The model under review builds one solid part; all positions refer to its coordinate system, in mm. Face numbers are marked on the shaded views. A direction names the side the tool comes from. Coordinates: 2 decimals unless noted, no trailing zeros. Write each loop counter-clockwise with the first axis right and the second up, starting at its lowest first coordinate (ties: lowest second). Pieces come first, ordered by that corner, then holes.
Autodesk Inventor part; units mm, degrees
ref_plane "YZ Plane" through (0, 0, 0) normal (1, 0, 0) x (0, 1, 0)
ref_plane "XZ Plane" through (0, 0, 0) normal (0, 1, 0) x (-1, 0, 0)
ref_plane "XY Plane" through (0, 0, 0) normal (0, 0, 1) x (1, 0, 0)
sketch "스케치1" plane through (0, 0, 0) normal (0, 0, 1) x (1, 0, 0)
  circle A0 centre (-5.4019, -4.5) radius 1.35
  circle A1 centre (5.4019, -4.5) radius 1.35
  circle A2 centre (-10.2056, -4.5) radius 1.35
  circle A3 centre (10.2056, -4.5) radius 1.35
  line L0 (-3.0587, -2.4) -> (-3.0587, -6.5)
  arc A4 (-3.0587, -6.5) -> (-4.0587, -7.5) centre (-3.0587, -7.5) ccw
  line L1 (-4.0587, -7.5) -> (-12.6075, -7.5)
  line L2 (-12.6075, -7.5) -> (-12.6075, 7.5)
  line L3 (-12.6075, 7.5) -> (-17.6, 13.3735)
  line L4 (-17.6, 13.3735) -> (-17.6, 24.9)
  line L5 (-17.6, 24.9) -> (-12.2, 24.9)
  line L6 (-12.2, 24.9) -> (-12.2, 14.7038)
  arc A5 (-12.2, 14.7038) -> (-10.2, 12.7038) centre (-10.2, 14.7038) ccw
  line L7 (-10.2, 12.7038) -> (0, 12.7038)
  line L8 (0, 12.7038) -> (5.5223, 12.4914)
  line L9 (5.5223, 12.4914) -> (10.5959, 12.4914)
  arc A6 (10.5959, 12.4914) -> (12.5959, 14.4914) centre (10.5959, 14.4914) ccw
  line L10 (12.5959, 14.4914) -> (12.5959, 24.9)
  line L11 (12.5959, 24.9) -> (17.6, 24.9)
  line L12 (17.6, 24.9) -> (17.6, 13.3735)
  line L13 (17.6, 13.3735) -> (12.6075, 7.5)
  line L14 (12.6075, 7.5) -> (12.6075, -7.5)
  line L15 (12.6075, -7.5) -> (4.1413, -7.5)
  arc A7 (4.1413, -7.5) -> (3.1413, -6.5) centre (3.1413, -7.5) ccw
  line L16 (3.1413, -6.5) -> (3.1413, -2.4)
  arc A8 (3.1413, -2.4) -> (2.1413, -1.4) centre (3.1413, -1.4) ccw
  line L17 (2.1413, -1.4) -> (-2.0587, -1.4)
  arc A9 (-2.0587, -1.4) -> (-3.0587, -2.4) centre (-3.0587, -1.4) ccw
  circle A10 centre (-8.5, 10.1) radius 1.45
  circle A11 centre (-15, 16.4) radius 1.45
  circle A12 centre (15, 16.4) radius 1.45
  circle A13 centre (8.5, 10.1) radius 1.45
  line L18 (12.6075, -7.5) -> (-12.6075, -7.5)
  line L19 (-12.6075, -7.5) -> (-12.6075, -1.5)
  line L20 (-12.6075, -1.5) -> (12.6075, -1.5)
  line L21 (12.6075, -1.5) -> (12.6075, -7.5)
  line L22 (3.1413, -1.4) -> (3.0413, -1.4)
  line L23 (3.0413, -1.4) -> (3.0413, -1.5)
  line L24 (3.0413, -1.5) -> (3.1413, -1.5)
  line L25 (3.1413, -1.5) -> (3.1413, -1.4)
  line L26 (3.0413, -1.5) -> (-2.9587, -1.5)
  line L27 (-2.9587, -1.5) -> (-2.9587, -7.5)
  line L28 (-2.9587, -7.5) -> (3.0413, -7.5)
  line L29 (3.0413, -7.5) -> (3.0413, -1.5)
  point P0 (0, 0)
  point P1 (12.6075, -1.5)
  dimension "d0" = 6
  dimension "d1" = 0.1
  dimension "d2" = 0.1
  dimension "d3" = 6
  dimension "d4" = 6
extrude "돌출1" add sketch "스케치1" along normal blind 30 contours A9 L20 L27 L18 A4 L0 | L0 A4 L1 L2 L20 A9 | L20 L29 L18 L27 | L20 A8 L16 A7 L18 L29 | L20 L14 L15 A7 L16 A8
sketch "스케치3" plane through (-12.6075, -7.5, 0) normal (0, -1, 0) x (1, 0, 0)
  line L0 (15.7488, 36) -> (15.7488, 30)
  line L1 (9.5488, 36) -> (9.5488, 30)
  line L2 (15.7488, 36) -> (15.6488, 36)
  line L3 (15.6488, 36) -> (15.6488, 35.9)
  line L4 (15.6488, 35.9) -> (15.7488, 35.9)
  line L5 (15.7488, 35.9) -> (15.7488, 36)
  line L6 (15.6488, 35.9) -> (9.6488, 35.9)
  line L7 (9.6488, 35.9) -> (9.6488, 29.9)
  line L8 (9.6488, 29.9) -> (15.6488, 29.9)
  line L9 (15.6488, 29.9) -> (15.6488, 35.9)
  line L10 (15.6488, 35.9) -> (9.6488, 35.9)
  line L11 (9.6488, 35.9) -> (9.6488, 36)
  line L12 (9.6488, 36) -> (15.6488, 36)
  line L13 (15.6488, 36) -> (15.6488, 35.9)
  line L14 (0, 30) -> (25.215, 30)
  line L15 (0, 0) -> (0, 30)
  line L16 (0, 15) -> (25.215, 15)
  line L17 (25.215, 0) -> (25.215, 30)
  line L18 (15.7488, -6) -> (15.7488, 0)
  line L19 (9.5488, -6) -> (9.5488, 0)
  line L20 (15.7488, -6) -> (15.6488, -6)
  line L21 (15.6488, -6) -> (15.6488, -5.9)
  line L22 (15.6488, -5.9) -> (15.7488, -5.9)
  line L23 (15.7488, -5.9) -> (15.7488, -6)
  line L24 (15.6488, -5.9) -> (9.6488, -5.9)
  line L25 (9.6488, -5.9) -> (9.6488, 0.1)
  line L26 (9.6488, 0.1) -> (15.6488, 0.1)
  line L27 (15.6488, 0.1) -> (15.6488, -5.9)
  line L28 (15.6488, -5.9) -> (9.6488, -5.9)
  line L29 (9.6488, -5.9) -> (9.6488, -6)
  line L30 (9.6488, -6) -> (15.6488, -6)
  line L31 (15.6488, -6) -> (15.6488, -5.9)
  line L32 (0, 0) -> (25.215, 0)
  point P0 (12.6075, 0)
  dimension "d11" = 0.1
  dimension "d12" = 0.1
  dimension "d13" = 6
  dimension "d14" = 6
extrude "돌출2" add sketch "스케치3" against normal blind 6 contours L9 L14 L7 L6 | L9 L8 L7 L14 | L32 L25 L26 L27 | L27 L24 L25 L32 | L21 L30 L29 L24
sketch "스케치7" plane through (-12.6075, -7.5, 0) normal (0, -1, 0) x (1, 0, 0)
  line L0 (0, 30) -> (9.6488, 30)
  line L1 (0, 0) -> (0, 30)
  line L2 (0, 0) -> (9.6488, 0)
  line L3 (9.6488, 0) -> (9.6488, -6)
  line L4 (9.6488, -6) -> (15.6488, -6)
  line L5 (15.6488, -6) -> (15.6488, 0)
  line L6 (15.6488, 0) -> (25.215, 0)
  line L7 (25.215, 0) -> (25.215, 30)
  line L8 (15.6488, 30) -> (25.215, 30)
  line L9 (15.6488, 30) -> (15.6488, 35.9)
  line L10 (15.6488, 35.9) -> (9.6488, 35.9)
  line L11 (9.6488, 35.9) -> (9.6488, 30)
  line L12 (0, 0) -> (0, 30)
  line L13 (0, 0) -> (-2.3925, 0)
  line L14 (-2.3925, 0) -> (-2.3925, 30)
  line L15 (-2.3925, 30) -> (0, 30)
  line L16 (0, 30) -> (0, 0)
  line L17 (12.6075, 0) -> (12.6075, 30)
  line L18 (25.215, 0) -> (25.215, 30)
  line L19 (25.215, 0) -> (25.215, 30)
  line L20 (25.215, 0) -> (27.6075, 0)
  line L21 (27.6075, 0) -> (27.6075, 30)
  line L22 (27.6075, 30) -> (25.215, 30)
  line L23 (25.215, 30) -> (25.215, 0)
  dimension "d26" = 2.3925
extrude "돌출6" add sketch "스케치7" against normal blind 6 contours L1 L13 L14 L15 | L22 L21 L20 L7
sketch "스케치8" plane through (-15, -7.5, 0) normal (-1, 0, 0) x (0, 0, 1)
  line L0 (0, 0) -> (30, 0)
  line L1 (15, 0) -> (15, 6)
  line L2 (30, 6) -> (0, 6)
  line L3 (15, 6) -> (12, 6)
  line L4 (12, 6) -> (12, 0)
  line L5 (12, 0) -> (15, 0)
  line L6 (15, 0) -> (15, 6)
  line L7 (15, 0) -> (18, 0)
  line L8 (18, 0) -> (18, 6)
  line L9 (18, 6) -> (15, 6)
  line L10 (15, 6) -> (15, 0)
  point P0 (0, 7.5)
  dimension "d29" = 3
  dimension "d30" = 3
extrude "돌출7" add sketch "스케치8" along normal blind 6
sketch "스케치9" plane through (-2.9587, -1.5, -6) normal (0, 1, 0) x (1, 0, 0)
  line L0 (6, -36) -> (17.9587, -36)
  line L1 (17.9587, -36) -> (17.9587, -6)
  line L2 (17.9587, -6) -> (6, -6)
  line L3 (6, -6) -> (6, 0)
  line L4 (6, 0) -> (0, 0)
  line L5 (0, 0) -> (0, -6)
  line L6 (0, -6) -> (-12.0413, -6)
  line L7 (-12.0413, -6) -> (-12.0413, -18)
  line L8 (-12.0413, -18) -> (-18.0413, -18)
  line L9 (-18.0413, -24) -> (-18.0413, -18)
  line L10 (-12.0413, -24) -> (-18.0413, -24)
  line L11 (-12.0413, -24) -> (-12.0413, -36)
  line L12 (0, -36) -> (-12.0413, -36)
  line L13 (0, -36) -> (0, -41.9)
  line L14 (0, -41.9) -> (6, -41.9)
  line L15 (6, -41.9) -> (6, -36)
  line L16 (2.9587, -6) -> (2.9587, -36)
  line L17 (17.9587, -18) -> (23.9587, -18)
  line L18 (23.9587, -24) -> (23.9587, -18)
  line L19 (17.9587, -24) -> (23.9587, -24)
extrude "돌출8" add sketch "스케치9" against normal blind 6 contours L1 L17 L18 L19
sketch "스케치10" plane through (15, -7.5, 0) normal (1, 0, 0) x (0, 0, -1)
  point P0 (0, 7.5)
sketch "스케치11" plane through (15, -7.5, 0) normal (1, 0, 0) x (0, 0, -1)
  circle A0 centre (-4.8357, 3) radius 1.35
  circle A1 centre (-9.6394, 3) radius 1.35
  circle A2 centre (-25.2469, 3) radius 1.35
  circle A3 centre (-20.4431, 3) radius 1.35
  point P0 (0, 7.5)
extrude "돌출9" cut sketch "스케치11" against normal through all
properties part number "부품78"
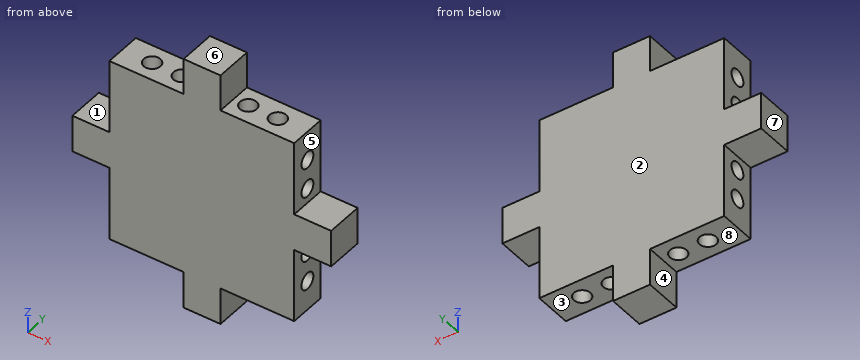
Item 1: To check wall thickness, follow line 1 along Z through (x, y) = (11.75, -4.5); line 2 along Z through (x, y) = (3, -4.5); line 3 along X through (y, z) = (-4.5, 23.3). State the ranges of each line that lie inside material, in increasing order.
Solved:
line 1: z = 0 to 3.49, 6.19 to 8.29, 10.99 to 19.09, 21.79 to 23.9, 26.6 to 30
line 2: z = -6 to 3.49, 6.19 to 8.29, 10.99 to 19.09, 21.79 to 23.9, 26.6 to 35.9
line 3: x = -15 to -11.56, -8.86 to -6.75, -4.05 to 4.05, 6.75 to 8.86, 11.56 to 15
Item 2: Machinability: for the marked faces 1, 2, 3, 4 and 5, which of the approach directions +Z, -Z, +X, -X, +Y, -Y give a long, thin tool a straight path to every point of the face, cutting with its end or side? Answer none if there is none.
Solved:
face 1: +Z, -X, +Y, -Y
face 2: +Z, -Z, +X, -X, +Y
face 3: -Z, +X, +Y, -Y
face 4: -Z, -X, +Y, -Y
face 5: +Z, +X, +Y, -Y
Item 3: For pin 1 (3.5 mm diameter, centred on y = -4.5, z = 9.64, fed in from +X); pin 2 (12 mm diameter, centred on x = 9.5, z = 30.5, fed in from -Y); pin 3 (3 mm diameter, centred on y = -4.5, z = 20.44, fed in from -X), all flat-tipped, find the tip position at first contact; note any pin that passes through.
Solved:
pin 1: stops at x = 15
pin 2: stops at y = -7.5
pin 3: stops at x = -15
Item 4: Mouldability with a two-part tool opening along Z and no side actions: class the marked faces 6, 7 and 8 as pulls with the +Z half, pulls with the -Z half, needs draft (parallel to the pull), parting line crosses it, or undercut.
Solved:
face 6: pulls with the +Z half
face 7: needs draft
face 8: pulls with the -Z half
Item 5: Take a section at C-C, the plane y = -4.5. Count the separate pieces of the cut face and the enclosed holes in it, plus the area to 3 significant figures.
Solved:
separate pieces: 25
enclosed holes: 0
area: 512 mm2
Item 6: Take a section at A-A, the plane x = 0. Write out the cut boundary in (y, z), plus the area to 3 significant figures.
Solved:
outline: (-7.5, -6) - (-1.5, -6) - (-1.5, 35.9) - (-7.5, 35.9) - close; hole circle Ø2.7 at (-4.5, 4.84); hole circle Ø2.7 at (-4.5, 9.64); hole circle Ø2.7 at (-4.5, 20.44); hole circle Ø2.7 at (-4.5, 25.25)
area: 228 mm2
Item 7: Take a section at B-B, the plane z = 29. Write out the cut boundary in (x, y), plus the area to 3 significant figures.
Solved:
outline: (-15, -7.5) - (15, -7.5) - (15, -1.5) - (-15, -1.5) - close; hole circle Ø2.7 at (-10.21, -4.5); hole circle Ø2.7 at (-5.4, -4.5); hole circle Ø2.7 at (5.4, -4.5); hole circle Ø2.7 at (10.21, -4.5)
area: 157 mm2
